```python
from build123d import *

# Parameters (mm, degrees)
F0_W           = 101.6
F0_H           = 38.1
F1_DEPTH       = 12.7
F2_W           = 38.1
F2_H           = 12.7
F3_DEPTH       = 12.7
F4_D           = 11.90625
F4_CBORE_D     = 25.4
F4_CBORE_DEPTH = 6.35
F5_W           = 38.0556955934
F5_H           = 3.175
F6_DEPTH       = 38.101
F8_D           = 10.0838
F9_R           = 3.17499
F10_R          = 3.17499


# Not quite as in the source:
# - a fillet or chamfer is up to 0.001 mm smaller than in the source, because OpenCascade refuses the exact size
# - a length typed as a fraction of an inch, garbled in the dataset ("3 / 203.2 mm" for 3/8 in), is restored


with BuildPart() as f1:
    # F0 (on Top) → F1 (new body)
    with BuildSketch(Plane.XY):
        with Locations((50.8, 19.05)):
            Rectangle(F0_W, F0_H)
    extrude(amount=F1_DEPTH)

    # F2 (on face) → F3 (join)
    with BuildSketch(Plane.XZ):
        with BuildLine():
            Line((31.75, 38.1), (31.75, 12.7))
            Line((31.75, 12.7), (69.85, 12.7))
            Line((69.85, 12.7), (69.85, 38.1))
            ThreePointArc((69.85, 38.1), (50.8, 57.15), (31.75, 38.1))
        make_face()
        with Locations((50.8, 6.35)):
            Rectangle(F2_W, F2_H)
    extrude(amount=-F3_DEPTH)

    # F4 (through all)
    with Locations(Plane.XZ):
        with Locations((50.8, 38.1)):
            CounterBoreHole(F4_D / 2, F4_CBORE_D / 2, F4_CBORE_DEPTH)

    # F5 (on face) → F6 (cut, through all)
    with BuildSketch(Plane(origin=(0, 38.1, 0), x_dir=(-1, 0, 0), z_dir=(0, 1, 0))):
        with Locations((-50.798330456, 1.5875)):
            Rectangle(F5_W, F5_H)
    extrude(amount=-F6_DEPTH, mode=Mode.SUBTRACT)

    # F8 (through all)
    with Locations(Plane.XY.offset(12.7)):
        with Locations((12.7, 25.4), (88.9, 25.4)):
            Hole(F8_D / 2)

    # F9 (radius 3.175 in the source; OpenCascade refuses exactly that, so slightly less here)
    f9_edges = [f1.edges().sort_by_distance(p)[0] for p in [
        (101.6, 38.1, 6.35),
        (0, 38.1, 6.35),
        (0, 0, 6.35),
        (101.6, 0, 6.35),
        (31.770483, 19.05, 3.175),
        (69.826178, 19.05, 3.175),
    ]]
    fillet(f9_edges, radius=F9_R)

    # F10 (radius 3.175 in the source; OpenCascade refuses exactly that, so slightly less here)
    f10_edges = [f1.edges().sort_by_distance(p)[0] for p in [
        (17.462495, 0, 12.7),
        (50.8, 38.1, 12.7),
        (0, 19.05, 12.7),
        (84.137505, 0, 12.7),
        (101.6, 19.05, 12.7),
        (69.85, 6.35, 12.7),
        (50.8, 0, 57.15),
        (50.8, 12.7, 57.15),
        (69.85, 12.7, 25.4),
        (50.8, 12.7, 12.7),
        (31.75, 6.35, 12.7),
        (31.75, 12.7, 25.4),
        (31.75, 0, 25.4),
        (69.85, 0, 25.4),
    ]]
    fillet(f10_edges, radius=F10_R)


solid = f1.part
```
Read the model definition and answer for the solid it produces. Units are mm, in the model's axes. A direction names the side the tool comes from. Coordinates: 2 decimals unless noted, no trailing zeros. Order: outer loops, then holes, each group sorted by start corner. A loop starts at its lowest first (then second) coordinate and runs counter-clockwise, first axis right, second up. Notation, with made-up numbers: (60, 83) - (85, 83) arc R22 cw to (85, 118) - close; hole circle Ø11 at (-23, -22.5). An arc over 180 degrees is marked (long way). Answer as a JSON object with one key per item and string values. Group by question number.
Item 1: A tool of negligible diameter and unlimited length cuts with its end or side. For faces 4 (the face through (16.05, 0.91, 11.75)), 5 (the face through (41.44, 3.131, 46.683)), 6 (the face through (68.94, 11.75, 27.14)), from which of +Z, -Z, +X, -X, +Y, -Y can it reach the whole face along a straight path? Write none if from no direction.
Item 2: The mould has two halves that part along X. Classify faces 1 (the face through (68.9, 0.91, 27.14)), 2 (the face through (50, 23, 12.7)), 3 (the face through (51, 19, 3.175)): +X half, -X half, draft (parallel to the pull), parting line (faces both ways), or undercut.
Item 3: Flat-ended cylindrical pins translate along their axes: P1, Ø9.5, axis at x = 46.5, y = 27.5, coming from the -Z side (3 decimals); P2, Ø4, axis at x = 59.5, z = 39.5, coming from the +Y side; P3, Ø6, axis at x = 35.5, y = 29, coming from the -Z side. Find the tip coordinate at first contact, or state that the pin passes through.
Item 4: Section C-C (z = 34) is taken. Give the vertices of the cut face in (x, y) (3 decimals).
Item 5: Consider probe 1 along Y at (x, z) = (12.7, 3.5); probe 2 along Z at (x, y) = (56, 20) (3 decimals); probe 3 along X at (y, z) = (10, 31.5). Determine where each line is inside the solid, lowest interval first. Write a range as from..to.
Item 6: Section D-D (x = 88.9) is taken. Give the vertices of the cut face in (y, z) (3 decimals).
Item 7: Section A-A (x = 50.8) is taken. Give the vertices of the cut face in (y, z) (3 decimals).
Results are:
{
 "1": {"face 4": "+Z, -X, -Y", "face 5": "-Y", "face 6": "+Z, +X, +Y"},
 "2": {"face 1": "+X half", "face 2": "draft", "face 3": "undercut"},
 "3": {"P1": "stops at z = 3.175", "P2": "stops at y = 12.7", "P3": "stops at z = 2.02"},
 "4": {"outline": "(31.75, 3.175) arc R3.175 ccw to (34.925, 0) - (38.78, 0) - (38.78, 6.35) - (46.484, 6.35) - (46.484, 12.7) - (34.925, 12.7) arc R3.175 ccw to (31.75, 9.525) - close; (55.116, 6.35) - (62.82, 6.35) - (62.82, 0) - (66.675, 0) arc R3.175 ccw to (69.85, 3.175) - (69.85, 9.525) arc R3.175 ccw to (66.675, 12.7) - (55.116, 12.7) - close"},
 "5": {"probe 1": "y = 0..20.36, 30.44..38.1", "probe 2": "z = 3.175..12.7", "probe 3": "x = 31.79..69.81"},
 "6": {"outline": "(0, 0) - (20.358, 0) - (20.358, 12.7) - (3.175, 12.7) arc R3.175 ccw to (0, 9.525) - close; (30.442, 0) - (38.1, 0) - (38.1, 9.525) arc R3.175 ccw to (34.925, 12.7) - (30.442, 12.7) - close"},
 "7": {"outline": "(0, 3.175) - (38.1, 3.175) - (38.1, 9.525) arc R3.175 ccw to (34.925, 12.7) - (15.875, 12.7) arc R3.175 cw to (12.7, 15.875) - (12.7, 32.147) - (6.35, 32.147) - (6.35, 25.4) - (0, 25.4) - close; (0, 50.8) - (6.35, 50.8) - (6.35, 44.053) - (12.7, 44.053) - (12.7, 53.975) arc R3.175 ccw to (9.525, 57.15) - (3.175, 57.15) arc R3.175 ccw to (0, 53.975) - close"}
}
